Work out the finished part from the listing and answer in its coordinate system (mm). Face numbers are marked on the shaded views. A direction names the side the tool comes from. Round coordinates to 2 decimals unless told otherwise and drop trailing zeros. Write each loop counter-clockwise with the first axis right and the second up, starting at its lowest first coordinate (ties: lowest second). Pieces come first, ordered by that corner, then holes. Notation, with made-up numbers: (-38, 32) -> (-2, 32) arc R17 ccw to (-2, 50) -> close; hole circle Ø11 at (79, 58.5). An arc over 180 degrees is marked (long way). One line per item, written item: value.
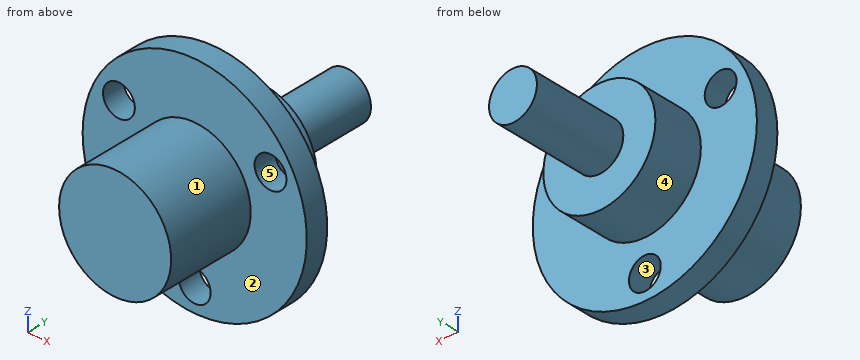
```python
from build123d import *

# Parameters (mm, degrees)
SKETCH2_R          = 1.5875
CUT_EXTRUDE1_DEPTH = 12.176
CIRPATTERN1_COUNT  = 3


with BuildPart() as part:
    # Sketch1 → Revolve1 (revolve)
    with BuildSketch(Plane.XY):
        Polygon((-5.588, 0), (-5.588, 8.89), (-11.176, 8.89), (-11.176, 11.176), (-5.588, 11.176), (-5.588, 16.256), (-2.3876, 16.256), (-2.3876, 25.908), (0, 25.908), (0, 0), align=None)
    revolve(axis=Axis((0, 25.908, 0), (0, -1, 0)))

    # Sketch2 → Cut-Extrude1 (cut, through all)
    with BuildSketch(Plane(origin=(0, 11.176, 0), x_dir=(1, 0, 0), z_dir=(0, 1, 0))):
        with Locations((0, 8.7249)):
            Circle(SKETCH2_R)
    cut_extrude1 = extrude(amount=-CUT_EXTRUDE1_DEPTH, mode=Mode.SUBTRACT)

    # CirPattern1: Cut-Extrude1 ×3 about axis
    cirpattern1_axis = Axis((0, 0, 0), (0, 1, 0))
    for i in range(1, CIRPATTERN1_COUNT):
        add(cut_extrude1.rotate(cirpattern1_axis, i * 360 / CIRPATTERN1_COUNT), mode=Mode.SUBTRACT)


solid = part.part
```
(1) Find section A-A on x = 0. Give the vertices of the cut face in (y, z), plus the area to 3 significant figures.
Reported:
outline: (0, -5.59) -> (8.89, -5.59) -> (8.89, -7.14) -> (11.18, -7.14) -> (11.18, -5.59) -> (16.26, -5.59) -> (16.26, -2.39) -> (25.91, -2.39) -> (25.91, 2.39) -> (16.26, 2.39) -> (16.26, 5.59) -> (11.18, 5.59) -> (11.18, 11.18) -> (8.89, 11.18) -> (8.89, 5.59) -> (0, 5.59) -> close; (8.89, -11.18) -> (11.18, -11.18) -> (11.18, -10.31) -> (8.89, -10.31) -> close
area: 246 mm2
(2) Find section D-D on x = -6.75. Give the vertices of the cut face in (y, z), plus the area to 3 significant figures.
Reported:
outline: (8.89, -8.91) -> (11.18, -8.91) -> (11.18, 2.99) -> (8.89, 2.99) -> close; (8.89, 5.73) -> (11.18, 5.73) -> (11.18, 8.91) -> (8.89, 8.91) -> close
area: 34.5 mm2
(3) A tool of negligible diameter and unlimited length cuts with its end or side. For the marked faces 4 and 5, from which of +Z, -Z, +X, -X, +Y, -Y can it reach the whole face along a straight path? Write none if from no direction.
Reported:
face 4: +Y
face 5: +Y, -Y
(4) Find section C-C on y = 23.25. Give the vertices of the cut face in (x, z).
Reported:
outline: circle Ø4.78 at (0, 0)
(5) For a pull along X with two mould halves and no side action, classify the marked faces 1, 2 and 3 as pulls with the +X half, pulls with the -X half, needs draft (parallel to the pull), parting line crosses it, or undercut.
Reported:
face 1: parting line crosses it
face 2: needs draft
face 3: undercut
(6) Flat-ended cylindrical pins translate along their axes: pin 1 Ø5 at (x, z) = (5, -7.5) entering from -Y; pin 2 Ø10 at (y, z) = (13, -5) entering from +X; pin 3 Ø8 at (x, y) = (-1.5, 3) entering from -Z. Find the tip coordinate at first contact, or state that the pin passes through.
Reported:
pin 1: stops at y = 8.89
pin 2: stops at x = 11.17
pin 3: stops at z = -5.59
(7) Find section B-B on z = -4.5. Give the vertices of the cut face in (x, y), plus the area to 3 significant figures.
Reported:
outline: (-10.23, 8.89) -> (-3.31, 8.89) -> (-3.31, 0) -> (3.31, 0) -> (3.31, 8.89) -> (10.23, 8.89) -> (10.23, 11.18) -> (3.31, 11.18) -> (3.31, 16.26) -> (-3.31, 16.26) -> (-3.31, 11.18) -> (-10.23, 11.18) -> close
area: 139 mm2
(8) Consider probe 1 along Z at (x, y) = (0, 10.55); probe 2 along Y at (x, z) = (7.5, 7.5); probe 3 along X at (y, z) = (9, 0.25). Determine where each line is inside the solid, lowest interval first.
Reported:
probe 1: z = -11.18 to -10.31, -7.14 to 11.18
probe 2: y = 8.89 to 11.18
probe 3: x = -11.17 to 11.17
